Check sheet for the modelled part. Datum: model origin and axes. Units: mm. Face numbers are marked on the shaded views. A direction names the side the tool comes from. Round coordinates to 2 decimals unless told otherwise and drop trailing zeros. Order: outer loops, then holes, each group sorted by start corner. A loop starts at its lowest first (then second) coordinate and runs counter-clockwise, first axis right, second up. Notation, with made-up numbers: (38, 2) -> (64, 2) arc R32 ccw to (64, 33) -> close; hole circle Ø8 at (-37.5, 25). An arc over 180 degrees is marked (long way). Answer in a Markdown table with one row per item.
```python
from build123d import *

# Parameters (mm, degrees)
SKETCH1_R           = 12.5
BOSS_EXTRUDE1_DEPTH = 50
BOSS_EXTRUDE2_START = 15
SKETCH3_R           = 15.5
BOSS_EXTRUDE2_DEPTH = 10
CIRPATTERN1_COUNT   = 7
FILLET1_R           = 1


with BuildPart() as part:
    # Sketch1 → Boss-Extrude1 (new body)
    with BuildSketch(Plane(origin=(0, 0, 0), x_dir=(1, 0, 0), z_dir=(0, 1, 0))):
        Circle(SKETCH1_R)
    extrude(amount=BOSS_EXTRUDE1_DEPTH)

    # Sketch3 → Boss-Extrude2 (add)
    with BuildSketch(Plane(origin=(0, 0, 0), x_dir=(1, 0, 0), z_dir=(0, 1, 0)).offset(BOSS_EXTRUDE2_START)):
        with BuildLine():
            Line((-2.253835774, 56.947383215), (-2.253835774, 12.295130105))
            Line((-2.253835774, 12.295130105), (2.253835774, 12.295130105))
            Line((2.253835774, 12.295130105), (2.253835774, 56.947383215))
            ThreePointArc((2.253835774, 56.947383215), (0, 92.805720885), (-2.253835774, 56.947383215))
        make_face()
        with Locations((0, 74.805720885)):
            Circle(SKETCH3_R, mode=Mode.SUBTRACT)
    boss_extrude2 = extrude(amount=BOSS_EXTRUDE2_DEPTH)

    # CirPattern1: Boss-Extrude2 ×7 about axis
    cirpattern1_axis = Axis((0, 0, 0), (0, 1, 0))
    for i in range(1, CIRPATTERN1_COUNT):
        add(boss_extrude2.rotate(cirpattern1_axis, i * 360 / CIRPATTERN1_COUNT))

    # Fillet1
    fillet1_edges = [part.edges().sort_by_distance(p)[0] for p in [
        (-12.5, 0, 0),
    ]]
    fillet(fillet1_edges, radius=FILLET1_R)


solid = part.part
```
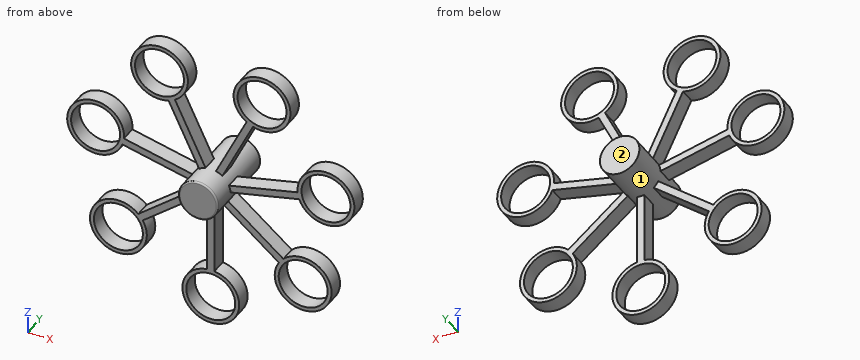
(1) Section check D-D on z = 24.5. Record the boundary of the cut face in (x, y).
Solutions:
| item | result |
|---|---|
| outline | (-89.13, 15) -> (-86.29, 15) -> (-86.29, 25) -> (-89.13, 25) -> close; (-59.57, 15) -> (-56.73, 15) -> (-56.73, 25) -> (-59.57, 25) -> close; (-14.3, 15) -> (-9.3, 15) -> (-9.3, 25) -> (-14.3, 25) -> close; (9.3, 15) -> (14.3, 15) -> (14.3, 25) -> (9.3, 25) -> close; (56.73, 15) -> (59.57, 15) -> (59.57, 25) -> (56.73, 25) -> close; (86.29, 15) -> (89.13, 15) -> (89.13, 25) -> (86.29, 25) -> close |
(2) Section check B-B on z = 72. Record the boundary of the cut face in (x, y), plus the area to 3 significant figures.
Solutions:
| item | result |
|---|---|
| outline | (-49.86, 15) -> (-47.26, 15) -> (-47.26, 25) -> (-49.86, 25) -> close; (-17.66, 15) -> (-15.06, 15) -> (-15.06, 25) -> (-17.66, 25) -> close; (15.06, 15) -> (17.66, 15) -> (17.66, 25) -> (15.06, 25) -> close; (47.26, 15) -> (49.86, 15) -> (49.86, 25) -> (47.26, 25) -> close |
| area | 104 mm^2 |
(3) Section check A-A on x = 0. Record the boundary of the cut face in (y, z).
Solutions:
| item | result |
|---|---|
| outline | (0, -11.5) arc R1 ccw to (1, -12.5) -> (15, -12.5) -> (15, -59.31) -> (25, -59.31) -> (25, -12.5) -> (50, -12.5) -> (50, 12.5) -> (1, 12.5) arc R1 ccw to (0, 11.5) -> close; (15, -92.81) -> (25, -92.81) -> (25, -90.31) -> (15, -90.31) -> close |
(4) Section check C-C on z = -71.5. Record the boundary of the cut face in (x, y), plus the area to 3 significant figures.
Solutions:
| item | result |
|---|---|
| outline | (-17.69, 15) -> (-15.14, 15) -> (-15.14, 25) -> (-17.69, 25) -> close; (15.14, 15) -> (17.69, 15) -> (17.69, 25) -> (15.14, 25) -> close |
| area | 51.0 mm^2 |
(5) Tool access check on the marked faces 1 and 2. Record the directions out of +Z, -Z, +X, -X, +Y, -Y that give a thin tool (end or side, any length) a straight path to the whole face; none if there is none.
Solutions:
| item | result |
|---|---|
| face 1 | none |
| face 2 | +Z, -Z, +X, -X, +Y |
(6) Depth check by flat-ended pin: pin 1 Ø11 at (x, z) = (40.5, 20) entering from +Y; pin 2 Ø5 at (y, z) = (39.5, -9.5) entering from +X; pin 3 Ø3 at (x, y) = (-9, 33) entering from -Z; pin 4 Ø18 at (x, z) = (-46, 21) entering from -Y. Enter the tip coordinate at first touch or a pass-through.
Solutions:
| item | result |
|---|---|
| pin 1 | through |
| pin 2 | x = 10.36 |
| pin 3 | z = -10 |
| pin 4 | y = 15 |
(7) Scan lines: probe 1 along Z at (x, y) = (1, 19.5); probe 2 along Z at (x, y) = (-36.5, 23.5); probe 3 along X at (y, z) = (19, 73). Record each from-to range of solid material in increasing order. Write a range as from..to.
Solutions:
| item | result |
|---|---|
| probe 1 | -92.78..-90.27, -59.34..12.46 |
| probe 2 | -31.99..-26.23, 6.02..10.64, 49.86..52.43, 82.36..84.94 |
| probe 3 | -49.56..-46.91, -18..-15.35, 15.35..18, 46.91..49.56 |
